For this review, take the finished solid that the model builds, in its own axes (mm). Face numbers are marked on the shaded views. Coordinates: 2 decimals unless noted, no trailing zeros. Write each loop counter-clockwise with the first axis right and the second up, starting at its lowest first coordinate (ties: lowest second). Pieces come first, ordered by that corner, then holes. Notation, with made-up numbers: (80.5, 61) -> (137.5, 61) arc R13 ccw to (137.5, 82) -> close; hole circle Ø1 at (-23.5, 9.5). An arc over 180 degrees is marked (long way). Put each result on its own line as item: value. Start each with the question number.
Item 1: The part is to be moulded in two halves that separate along Z. For the marked faces 1 and 2, say which applies: +Z half, -Z half, draft (parallel to the pull), parting line (faces both ways), or undercut.
Item 2: To check wall thickness, follow L1, parallel to Z at x = 14, y = 0.3; L2, parallel to X at y = 1.45, z = 6; L3, parallel to Z at x = -1.5, y = 0.8. State the ranges of each line that lie inside material, in increasing order.
Item 3: Insertion check: P1, Ø1.6, axis at x = 22, y = 1.5, coming from the -Z side; P2, Ø1, axis at y = 1, z = -21.5, coming from the -X side. Each pin has a flat end and moves straight along its axis. Give the tip position at first contact, or say it passes through.
Item 4: Consider section B-B on z = 14. Give the boundary of the cut face in (x, y).
Item 5: Consider section C-C on y = 1.45. Give the boundary of the cut face in (x, z), and give its area (3 significant figures).
Item 6: Consider section A-A on x = -7. Give the boundary of the cut face in (y, z), and give its area (3 significant figures).
Item 7: Consider section D-D on x = -15.75. Give the boundary of the cut face in (y, z).
```python
from build123d import *

# Parameters (mm, degrees)
BOSS_EXTRUDE1_DEPTH = 3
FILLET1_R           = 3
SKETCH2_R           = 1.6
SKETCH2_W           = 15
SKETCH2_H           = 29
SKETCH2_W_2         = 11
CUT_EXTRUDE1_DEPTH  = 3
SKETCH4_W           = 14
SKETCH4_H           = 29.4
CUT_EXTRUDE2_DEPTH  = 2


with BuildPart() as part:
    # Sketch1 → Boss-Extrude1 (new body)
    with BuildSketch(Plane(origin=(0, 0, 0), x_dir=(1, 0, 0), z_dir=(0, 1, 0))):
        Polygon((-20.75, 42), (-20.75, 0), (-25.75, 0), (-25.75, -42), (25.75, -42), (25.75, 0), (20.75, 0), (20.75, 42), align=None)
    extrude(amount=BOSS_EXTRUDE1_DEPTH)

    # Fillet1
    fillet1_edges = [part.edges().sort_by_distance(p)[0] for p in [
        (20.75, 1.5, -42),
        (25.75, 1.5, 0),
        (25.75, 1.5, 42),
        (-25.75, 1.5, 42),
        (-25.75, 1.5, 0),
        (-20.75, 1.5, -42),
    ]]
    fillet(fillet1_edges, radius=FILLET1_R)

    # Sketch2 → Cut-Extrude1 (cut)
    with BuildSketch(Plane(origin=(0, 3, 0), x_dir=(1, 0, 0), z_dir=(0, 1, 0))):
        with Locations(Location((-15.75, -35.907418342, 0), (0, 0, 270))):
            Circle(SKETCH2_R)
        with Locations((-12.5, -15.5)):
            Rectangle(SKETCH2_W, SKETCH2_H)
        with Locations((14.5, -15.5)):
            Rectangle(SKETCH2_W_2, SKETCH2_H)
    extrude(amount=-CUT_EXTRUDE1_DEPTH, mode=Mode.SUBTRACT)

    # Sketch4 → Cut-Extrude2 (cut)
    with BuildSketch(Plane.XZ):
        with Locations((2, 15.5)):
            Rectangle(SKETCH4_W, SKETCH4_H)
    extrude(amount=-CUT_EXTRUDE2_DEPTH, mode=Mode.SUBTRACT)


solid = part.part
```
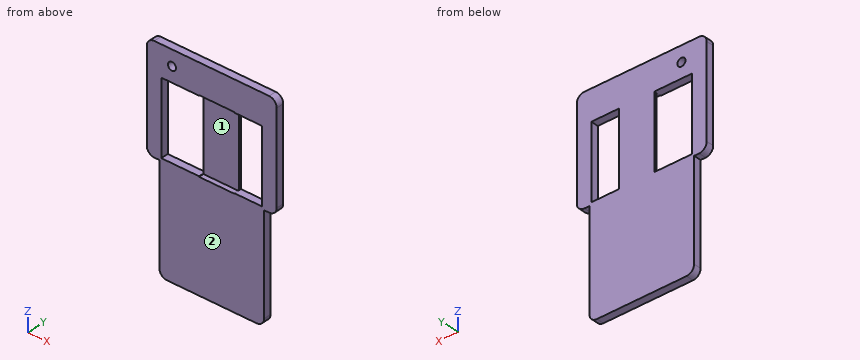
Return value:
1. face 1: undercut
1. face 2: draft
2. L1: -42 to 1, 30 to 42
2. L2: -25.75 to -20, 20 to 25.75
2. L3: -42 to 0.8, 30.2 to 42
3. P1: z = 0
3. P2: x = -20.75
4. outline: (-25.75, 0) -> (-20, 0) -> (-20, 3) -> (-25.75, 3) -> close; (-5, 2) -> (9, 2) -> (9, 3) -> (-5, 3) -> close; (20, 0) -> (25.75, 0) -> (25.75, 3) -> (20, 3) -> close
5. outline: (-25.75, 3) arc R3 ccw to (-22.75, 0) -> (-20.75, 0) -> (-20.75, -39) arc R3 ccw to (-17.75, -42) -> (17.75, -42) arc R3 ccw to (20.75, -39) -> (20.75, 0) -> (22.75, 0) arc R3 ccw to (25.75, 3) -> (25.75, 39) arc R3 ccw to (22.75, 42) -> (-22.75, 42) arc R3 ccw to (-25.75, 39) -> close; hole (-20, 1) -> (-5, 1) -> (-5, 0.8) -> (9, 0.8) -> (9, 1) -> (20, 1) -> (20, 30) -> (9, 30) -> (9, 30.2) -> (-5, 30.2) -> (-5, 30) -> (-20, 30) -> close; hole circle Ø3.2 at (-15.75, 35.91)
5. area: 2,720 mm^2
6. outline: (0, -42) -> (3, -42) -> (3, 1) -> (0, 1) -> close; (0, 30) -> (3, 30) -> (3, 42) -> (0, 42) -> close
6. area: 165 mm^2
7. outline: (0, -42) -> (3, -42) -> (3, 1) -> (0, 1) -> close; (0, 30) -> (3, 30) -> (3, 34.31) -> (0, 34.31) -> close; (0, 37.51) -> (3, 37.51) -> (3, 42) -> (0, 42) -> close
